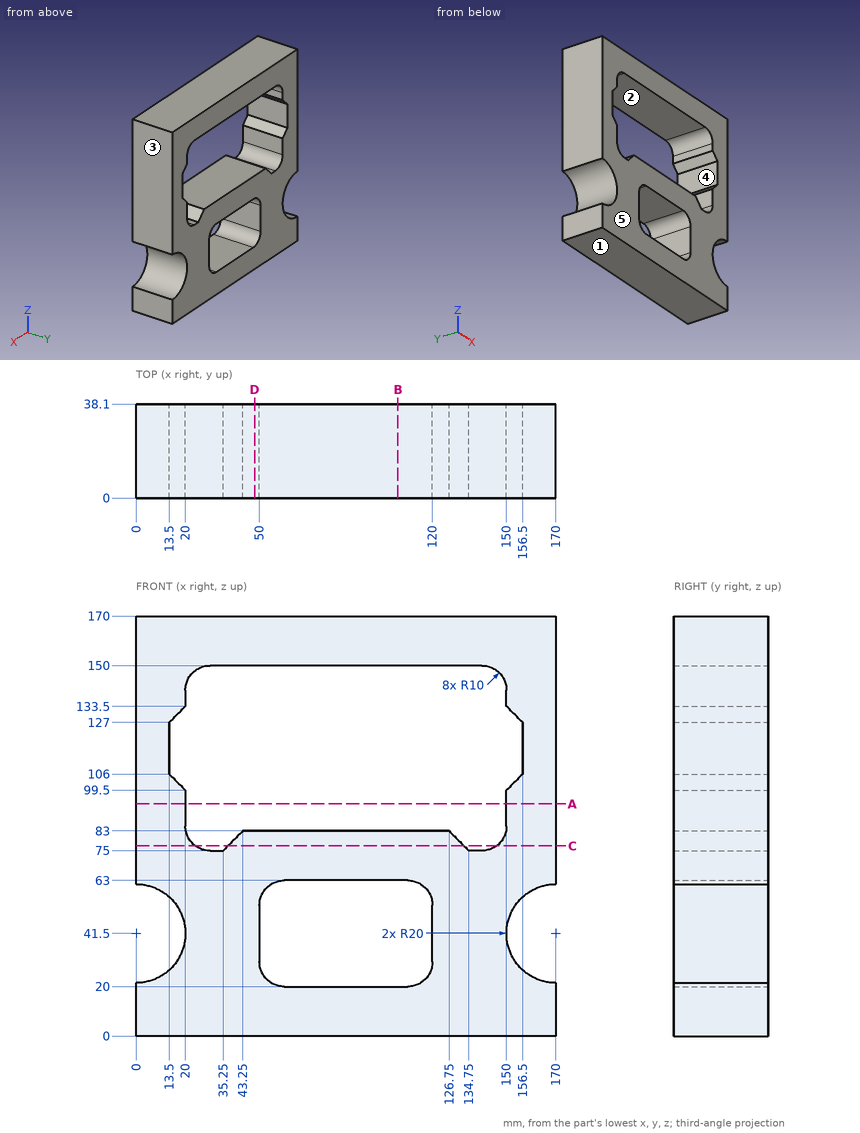
For this review, use the dimensioned drawing (mm, ordinates from the lowest corner) and the shaded views. A direction names the side the tool comes from. Give positions to 0.01 mm unless a question says otherwise; leave off trailing zeros. Order: outer loops, then holes, each group sorted by start corner. A loop starts at its lowest first (then second) coordinate and runs counter-clockwise, first axis right, second up. Notation, with made-up numbers: (45, 62) - (80, 62) arc R19 cw to (80, 71) - close; hole circle Ø11 at (-17, 75). An arc over 180 degrees is marked (long way). Write item = value, one per line. Start each with the question number.
Q1. We need section A-A on z = 94. State the section outline as (x, y) points.
Q2. We need section B-B on x = 106. State the section outline as (y, z) points, plus the area to 3 significant figures.
Q3. We need section C-C on z = 77. State the section outline as (x, y) points.
Q4. Clearance check with flat-ended pins moving along their axes: pin 1 Ø11.5 at (y, z) = (14.5, 44.5) entering from -X; pin 2 Ø11.5 at (y, z) = (16.5, 37) entering from +X. State where each tip first meets the part, or that it passes through.
Q5. We need section D-D on x = 48. State the section outline as (y, z) points.
Q6. To check wall thickness, follow L1, parallel to Z at x = 97.5, y = 4.5; L2, parallel to Z at x = 122.5, y = 17.5; L3, parallel to X at y = 10.5, z = 95. State the ranges of each line that lie inside material, in increasing order. Write a range as from..to.
Q7. Tool access review of the marked faces 4 and 5: name each direction out of +Z, -Z, +X, -X, +Y, -Y from which nothing blocks a thin tool from reaching the whole face with its end or side.
Q8. Mouldability with a two-part tool opening along Z and no side actions: class the marked faces 1, 2 and 3 as released by +Z, released by -Z, zero draft, split by the parting line, or undercut.
Working result:
q1.outline = (0, 0) - (20, 0) - (20, 38.1) - (0, 38.1) - close; (150, 0) - (170, 0) - (170, 38.1) - (150, 38.1) - close
q2.outline = (0, 0) - (38.1, 0) - (38.1, 20) - (0, 20) - close; (0, 63) - (38.1, 63) - (38.1, 83) - (0, 83) - close; (0, 150) - (38.1, 150) - (38.1, 170) - (0, 170) - close
q2.area = 2,290 mm²
q3.outline = (0, 0) - (24, 0) - (24, 38.1) - (0, 38.1) - close; (37.25, 0) - (132.75, 0) - (132.75, 38.1) - (37.25, 38.1) - close; (146, 0) - (170, 0) - (170, 38.1) - (146, 38.1) - close
q4.pin_1 = 17.98
q4.pin_2 = 152.83
q5.outline = (0, 0) - (38.1, 0) - (38.1, 83) - (0, 83) - close; (0, 150) - (38.1, 150) - (38.1, 170) - (0, 170) - close
q6.L1 = 0..20, 63..83, 150..170
q6.L2 = 0..83, 150..170
q6.L3 = 0..20, 150..170
q7.face_4 = +Y, -Y
q7.face_5 = +Z, -Z, +X, -X, -Y
q8.face_1 = released by -Z
q8.face_2 = undercut
q8.face_3 = zero draft
